from build123d import *

# Parameters (mm, degrees)
SM_BASE_FLANGE_1_DEPTH = 100
CUT_EXTRUDE_1_DEPTH    = 459.018558576


# Sheet-metal steps are written as plain solids
with BuildPart() as part:
    # Sketch 1 → 基体-法兰1 (new, symmetric)
    with BuildSketch(Plane(origin=(0, 0, 0), x_dir=(0, 0, -1), z_dir=(1, 0, 0))):
        with BuildLine():
            Line((270, -160), (8.396569497, -77.643364471))
            ThreePointArc((8.396569497, -77.643364471), (2.324227007, -73.295019402), (0, -66.197173462))
            Line((0, -66.197173462), (0, -6))
            ThreePointArc((0, -6), (-1.757359313, -1.757359313), (-6, 0))
            Line((-6, 0), (-415, 0))
            Line((-415, 0), (-415, 6))
            Line((-415, 6), (-6, 6))
            ThreePointArc((-6, 6), (2.485281374, 2.485281374), (6, -6))
            Line((6, -6), (6, -66.197173462))
            ThreePointArc((6, -66.197173462), (7.162113503, -69.746096432), (10.198284749, -71.920268967))
            Line((10.198284749, -71.920268967), (271.801715251, -154.276904496))
            Line((271.801715251, -154.276904496), (270, -160))
        make_face()
    extrude(amount=SM_BASE_FLANGE_1_DEPTH, both=True)

    # 草图4 → 切除-拉伸1 (cut, through all)
    with BuildSketch(Plane(origin=(0, 6, 0), x_dir=(1, 0, 0), z_dir=(0, 1, 0))):
        with BuildLine():
            Line((100, -415), (20, -358.983396943))
            Line((20, -358.983396943), (20, -265))
            ThreePointArc((20, -265), (-30, -215), (-80, -265))
            Line((-80, -265), (-80, -300))
            Line((-80, -300), (-100, -300))
            Line((-100, -300), (-100, -415))
            Line((-100, -415), (100, -415))
        make_face()
    extrude(amount=-CUT_EXTRUDE_1_DEPTH, mode=Mode.SUBTRACT)


solid = part.part
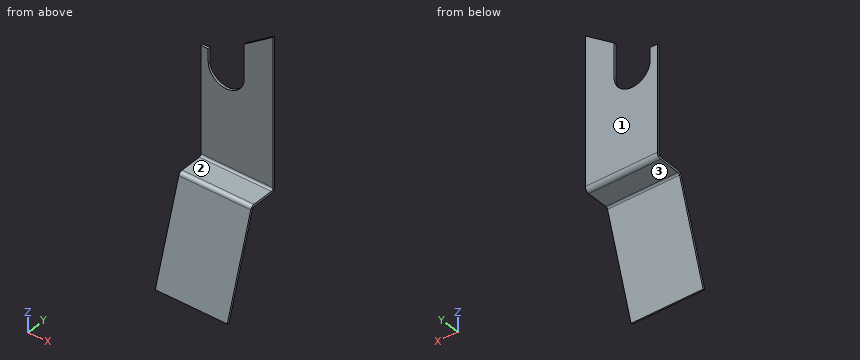
The listing builds one solid part. Answer for the finished solid, in the listing's coordinates (mm). Face numbers are marked on the shaded views. A direction names the side the tool comes from. Round coordinates to 2 decimals unless told otherwise and drop trailing zeros. Write each loop counter-clockwise with the first axis right and the second up, starting at its lowest first coordinate (ties: lowest second). Pieces come first, ordered by that corner, then holes. Notation, with made-up numbers: M 65,10 L 114,10 A23 cw 114,39 Z; hole C -7.75,79 d9. An arc over 180 degrees is marked long. Write each question's results on one line, items separated by ' | '. Start each with the question number.
(1) For the marked faces 1, 2 and 3, determine the directions among +Z, -Z, +X, -X, +Y, -Y from which every point of the face is accessible in a straight line to the end or side of a thin tool.
(2) The part is cut by section B-B, the plane y = -22.5. Write down the section's boundary in (x, z), and give its area (3 significant figures).
(3) The part is cut by section C-C, the plane z = -44.5. Write down the section's boundary in (x, y).
(4) The part is cut by section A-A, the plane x = -30. Write down the section's boundary in (y, z), and give its area (3 significant figures).
(5) Each of these flat-tipped pins is pushed along its axis until it touches: P1, Ø18, axis at x = -37, y = -30, coming from the -Z side; P2, Ø1.8, axis at y = 2.5, z = 335, coming from the -X side; P3, Ø1.5, axis at x = 57, y = -75, coming from the +Z side. Where does it stop, or does it pass through?
(6) Find the intervals of material crossed by line 1 (Y direction, x = -42, z = 19); line 2 (Z direction, x = 49, y = -9); line 3 (Y direction, x = 39.5, z = -190), in increasing order.
Worked answers:
1) face 1: +Z, -Z, +X, -X, +Y | face 2: +Z, +X, -X, -Y | face 3: -Z, +X, -X, +Y
2) outline: M -100,-6 L 100,-6 L 100,0 L -100,0 Z | area: 1,200 mm²
3) outline: M -100,-89.01 L 100,-89.01 L 100,-82.72 L -100,-82.72 Z
4) outline: M -160,-270 L -154.28,-271.8 L -71.92,-10.2 A6 cw -66.2,-6 L -6,-6 A12 ccw 6,6 L 6,215 L 0,215 L 0,6 A6 cw -6,0 L -66.2,0 A12 ccw -77.64,-8.4 Z | area: 3,410 mm²
5) P1: stops at z = -6 | P2: stops at x = 20 | P3: stops at z = -3.1
6) line 1: y = 0 to 6 | line 2: z = -6 to 0 | line 3: y = -134.81 to -128.52
